from build123d import *

# Parameters (mm, degrees)
F0_W     = 101.6
F0_H     = 101.6
F1_DEPTH = 6.35
F2_R     = 50.79999
F3_R     = 8.73125
F4_DEPTH = 25.4


# Not quite as in the source:
# - a fillet or chamfer is up to 0.001 mm smaller than in the source, because OpenCascade refuses the exact size


with BuildPart() as f1:
    # F0 (on Right) → F1 (new body, symmetric)
    with BuildSketch(Plane.YZ):
        with Locations((-50.8, 50.8)):
            Rectangle(F0_W, F0_H)
    extrude(amount=F1_DEPTH, both=True)

    # F2 (radius 50.8 in the source; OpenCascade refuses exactly that, so slightly less here)
    f2_edges = [f1.edges().sort_by_distance(p)[0] for p in [
        (0, -101.6, 101.6),
        (0, -101.6, 0),
    ]]
    fillet(f2_edges, radius=F2_R)

    # F3 (on face) → F4 (cut)
    with BuildSketch(Plane.YZ.offset(6.35)):
        with Locations((-50.8, 50.8)):
            Circle(F3_R)
    extrude(amount=-F4_DEPTH, mode=Mode.SUBTRACT)


solid = f1.part
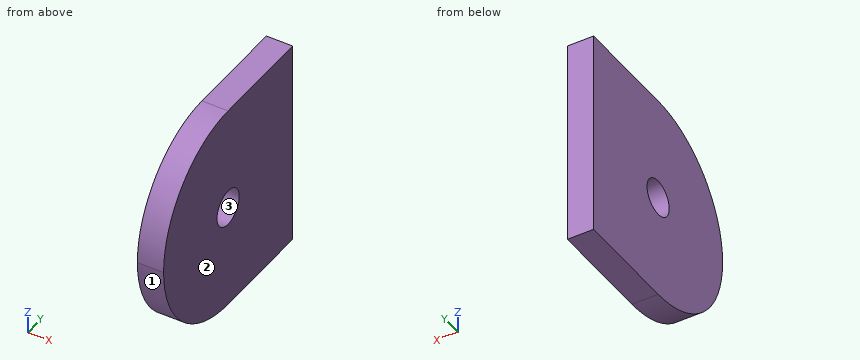
Could you check a few things on this model? Use its own coordinates, in mm. Face numbers are marked on the shaded views. Coordinates: 2 decimals unless noted, no trailing zeros. Loops run counter-clockwise (first coordinate to the right, second up) from the corner with the lowest first, then second, coordinate; pieces in that order, holes last. Notation, with made-up numbers: (52, 27) -> (79, 27) arc R22 ccw to (79, 42) -> close; hole circle Ø8 at (-18, 37). An arc over 180 degrees is marked (long way). Answer in a Markdown table with one row per item.
(1) If I drill on probe 1 along Z at (x, y) = (2.75, -50.8); probe 2 along Y at (x, z) = (-4.25, 47); probe 3 along Y at (x, z) = (-1.75, 56), over which ranges is the centre line in solid material (lowest first)?
Results found:
| item | result |
|---|---|
| probe 1 | z = 0 to 42.07, 59.53 to 101.6 |
| probe 2 | y = -101.46 to -58.66, -42.94 to 0 |
| probe 3 | y = -101.33 to -57.81, -43.79 to 0 |
(2) Imagine slicing it at D-D (y = -87). List the corners of the cut face in (x, z) for me, plus the area to 3 significant figures.
Results found:
| item | result |
|---|---|
| outline | (-6.35, 15.16) -> (6.35, 15.16) -> (6.35, 86.44) -> (-6.35, 86.44) -> close |
| area | 905 mm^2 |
(3) Imagine slicing it at B-B (z = 56.5). List the corners of the cut face in (x, y) for me, plus the area to 3 significant figures.
Results found:
| item | result |
|---|---|
| outline | (-6.35, -101.28) -> (6.35, -101.28) -> (6.35, -57.41) -> (-6.35, -57.41) -> close; (-6.35, -44.19) -> (6.35, -44.19) -> (6.35, 0) -> (-6.35, 0) -> close |
| area | 1,120 mm^2 |
(4) Thinking about a two-plate mould opening in Z: for the marked faces 1, 2 and 3, which applies, released by +Z, released by -Z, zero draft, split by the parting line, or undercut?
Results found:
| item | result |
|---|---|
| face 1 | released by -Z |
| face 2 | zero draft |
| face 3 | undercut |
(5) Imagine slicing it at C-C (z = 31). List the corners of the cut face in (x, y) for me, plus the area to 3 significant figures.
Results found:
| item | result |
|---|---|
| outline | (-6.35, -97.58) -> (6.35, -97.58) -> (6.35, 0) -> (-6.35, 0) -> close |
| area | 1,240 mm^2 |
(6) Will these pins go through, and if not, where does the flat tip stop? pin 1 Ø6 at (x, z) = (5, 56.5) entering from -Y; pin 2 Ø4 at (x, y) = (0.5, -77.5) entering from +Z.
Results found:
| item | result |
|---|---|
| pin 1 | stops at y = -101.53 |
| pin 2 | stops at z = 95.19 |
